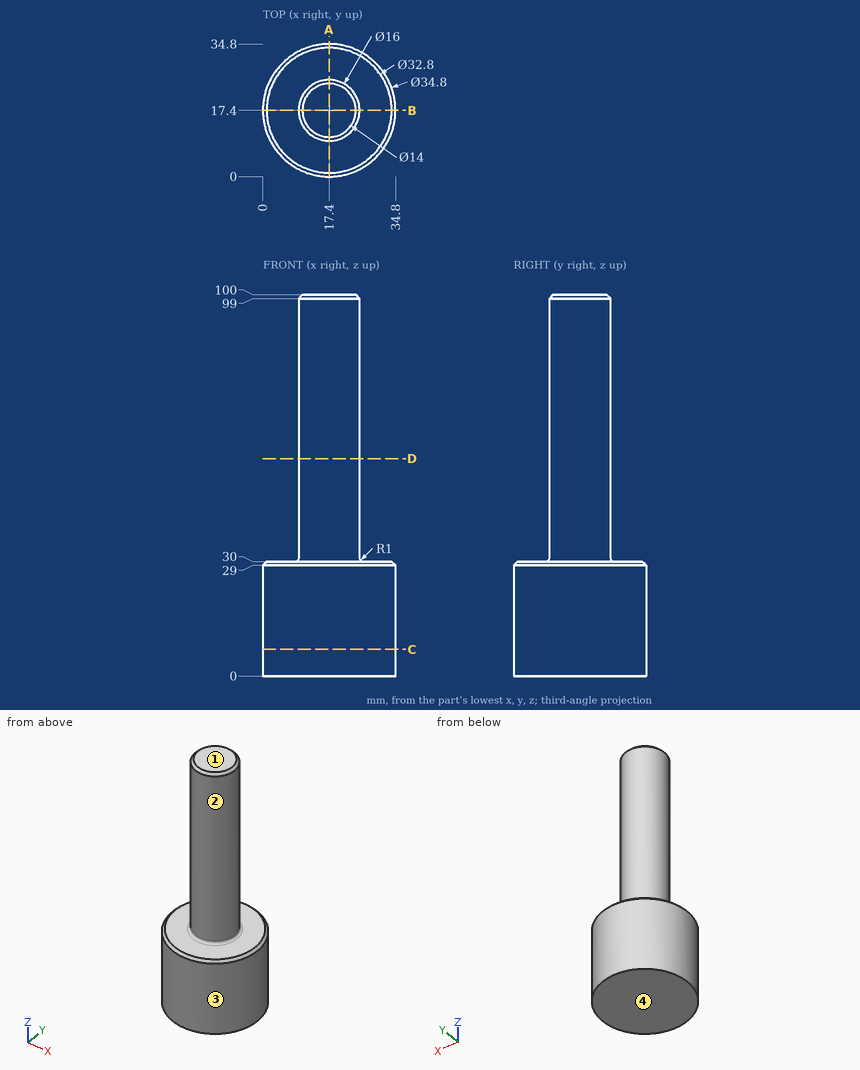
For this review, use the dimensioned drawing (mm, ordinates from the lowest corner) and the shaded views. A direction names the side the tool comes from. Coordinates: 2 decimals unless noted, no trailing zeros. Order: outer loops, then holes, each group sorted by start corner. A loop starts at its lowest first (then second) coordinate and runs counter-clockwise, first axis right, second up. Notation, with made-up numbers: (29.25, -37.5) -> (39.25, -37.5) arc R31 cw to (39.25, -1.5) -> close; hole circle Ø7 at (55.25, 70.5). An arc over 180 degrees is marked (long way). One line per item, written item: value. Start each with the question number.
Q1. Take a section at D-D, the plane z = 57. State the section outline as (x, y) points, then the cut area to 3 significant figures.
Q2. Insertion check: pin 1 Ø4 at (y, z) = (26, 70) entering from +X; pin 2 Ø3 at (y, z) = (6.5, 31) entering from +X; pin 3 Ø6 at (x, z) = (7, 82) entering from +Y. Each pin has a flat end and moves straight along its axis. Give the tip position at first contact, or say it passes through.
Q3. For probe 1 along Z at (x, y) = (10, 7.5); probe 2 along Z at (x, y) = (16.5, 25.5); probe 3 along X at (y, z) = (13, 73.5), list the stretches that pass through material, from the lowest coordinate up.
Q4. Tool access review of the marked faces 1 and 2: name each direction out of +Z, -Z, +X, -X, +Y, -Y from which nothing blocks a thin tool from reaching the whole face with its end or side.
Q5. Take a section at C-C, the plane z = 7. State the section outline as (x, y) points, then the cut area to 3 significant figures.
Q6. Take a section at A-A, the plane x = 17.4. State the section outline as (y, z) points, then the cut area to 3 significant figures.
Q7. Mouldability with a two-part tool opening along Y and no side actions: class the marked faces 3 and 4 as pulls with the +Y half, pulls with the -Y half, needs draft (parallel to the pull), parting line crosses it, or undercut.
Values follow:
1. outline: circle Ø16 at (17.4, 17.4)
1. area: 201 mm2
2. pin 1: stops at x = 21.92
2. pin 2: stops at x = 30.66
2. pin 3: stops at y = 20.44
3. probe 1: z = 0 to 30
3. probe 2: z = 0 to 30.47
3. probe 3: x = 10.72 to 24.08
4. face 1: +Z, +X, -X, +Y, -Y
4. face 2: +Z
5. outline: circle Ø34.8 at (17.4, 17.4)
5. area: 951 mm2
6. outline: (0, 0) -> (34.8, 0) -> (34.8, 29) -> (33.8, 30) -> (26.4, 30) arc R1 cw to (25.4, 31) -> (25.4, 99) -> (24.4, 100) -> (10.4, 100) -> (9.4, 99) -> (9.4, 31) arc R1 cw to (8.4, 30) -> (1, 30) -> (0, 29) -> close
6. area: 2,160 mm2
7. face 3: parting line crosses it
7. face 4: needs draft
